Can you work these out from the model? Positions are in its coordinate system, mm. Coordinates: 2 decimals unless noted, no trailing zeros. Write each loop counter-clockwise with the first axis right and the second up, starting at its lowest first coordinate (ties: lowest second). Pieces come first, ordered by that corner, then holes. Notation, with made-up numbers: (47, 82) - (86, 82) arc R34 ccw to (86, 112) - close; hole circle Ø11 at (-24, 13.5). An arc over 180 degrees is marked (long way). Use one line per item in the form item = value. Start each with the question number.
(1) If I drill on probe 1 along Y at (x, z) = (244, 1.5); probe 2 along Z at (x, y) = (-160.5, -0.25), over which ranges is the centre line in solid material (lowest first)? Write a range as from..to.
(2) If we section it at A-A on x = 216: Please give me the cut outline in (y, z), then the cut area to 3 significant figures.
(3) For pin 1 Ø1 at (x, y) = (-179, -9.5) entering from +Z; pin 2 Ø6.5 at (x, z) = (-184, 0) entering from -Y; pin 3 Ø1 at (x, y) = (55, -1) entering from -Z, each with a flat end and sliding along its axis, tell me the tip position at first contact or that it passes through.
(4) If we section it at B-B on x = -176: Please give me the cut outline in (y, z).
```python
from build123d import *

# Parameters (mm, degrees)
F0_R     = 12.5
F1_DEPTH = 352.5
F4_DEPTH = 4
F5_SIZE  = 1


with BuildPart() as f1:
    # F0 (on Right) → F1 (new body, symmetric)
    with BuildSketch(Plane.YZ):
        Circle(F0_R)
    extrude(amount=F1_DEPTH, both=True)

    # F3 (on offset) → F4 (cut)
    with BuildSketch(Plane.XZ.offset(12.5)):
        with BuildLine():
            ThreePointArc((-342.5, 4), (-346.5, 0), (-342.5, -4))
            Line((-342.5, -4), (-277.5, -4))
            ThreePointArc((-277.5, -4), (-273.5, 0), (-277.5, 4))
            Line((-277.5, 4), (-342.5, 4))
        make_face()
        with BuildLine():
            ThreePointArc((-194, 4), (-198, 0), (-194, -4))
            Line((-194, -4), (-164, -4))
            ThreePointArc((-164, -4), (-160, 0), (-164, 4))
            Line((-164, 4), (-194, 4))
        make_face()
        with BuildLine():
            ThreePointArc((254, 4), (250, 0), (254, -4))
            Line((254, -4), (284, -4))
            ThreePointArc((284, -4), (288, 0), (284, 4))
            Line((284, 4), (254, 4))
        make_face()
    extrude(amount=-F4_DEPTH, mode=Mode.SUBTRACT)

    # F5
    f5_edges = [f1.edges().sort_by_distance(p)[0] for p in [
        (352.5, -12.5, 0),
        (-352.5, -12.5, 0),
    ]]
    chamfer(f5_edges, length=F5_SIZE)


solid = f1.part
```
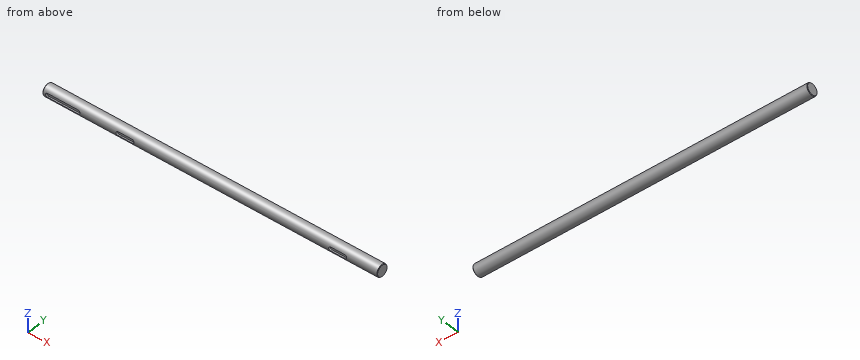
Reported:
q1.probe_1 = -12.41..12.41
q1.probe_2 = -12.5..12.5
q2.outline = circle Ø25 at (0, 0)
q2.area = 491 mm2
q3.pin_1 = 8.67
q3.pin_2 = -8.5
q3.pin_3 = -12.49
q4.outline = (-11.84, -4) arc R12.5 ccw (long way) to (-11.84, 4) - (-8.5, 4) - (-8.5, -4) - close
